Part model, mm, in its own coordinate system. Face numbers are marked on the shaded views. Round coordinates to 2 decimals unless told otherwise and drop trailing zeros. Loops run counter-clockwise (first coordinate to the right, second up) from the corner with the lowest first, then second, coordinate; pieces in that order, holes last.
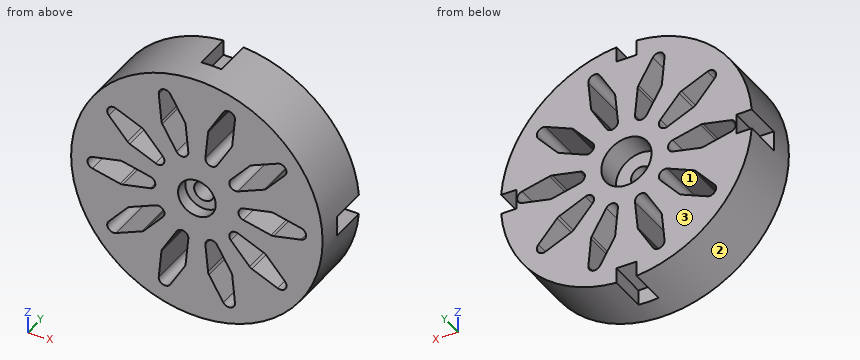
from build123d import *

# Parameters (mm, degrees)
SKETCH_1_R               = 20
SKETCH_1_R_2             = 4
EXTRUDE_1_DEPTH          = 10
SKETCH_4_R               = 20
EXTRUDE_2_DEPTH          = 6
SKETCH_5_R               = 1.6
CUT_EXTRUDE_2_DEPTH      = 5
CUT_EXTRUDE_2_DEPTH_BACK = 7
CUT_EXTRUDE_3_DEPTH      = 1
CUT_EXTRUDE_3_DEPTH_BACK = 11
SKETCH_8_W               = 3.2
SKETCH_8_H               = 5
SKETCH_8_W_2             = 5
SKETCH_8_H_2             = 3.2
CUT_EXTRUDE_4_DEPTH      = 6
SKETCH_9_R               = 3
CUT_EXTRUDE_5_DEPTH      = 2


with BuildPart() as part:
    # Эскиз1 → Бобышка-Вытянуть1 (new body)
    with BuildSketch(Plane(origin=(0, 0, 0), x_dir=(1, 0, 0), z_dir=(0, 1, 0))):
        Circle(SKETCH_1_R)
        Circle(SKETCH_1_R_2, mode=Mode.SUBTRACT)
    extrude(amount=EXTRUDE_1_DEPTH)

    # Эскиз4 → Бобышка-Вытянуть2 (add)
    with BuildSketch(Plane.XZ):
        Circle(SKETCH_4_R)
    extrude(amount=-EXTRUDE_2_DEPTH)

    # Эскиз5 → Вырез-Вытянуть2 (cut, two sides)
    with BuildSketch(Plane(origin=(0, 6, 0), x_dir=(1, 0, 0), z_dir=(0, 1, 0))) as cut_extrude_2_sk:
        Circle(SKETCH_5_R)
    extrude(amount=CUT_EXTRUDE_2_DEPTH, mode=Mode.SUBTRACT)
    extrude(cut_extrude_2_sk.sketch, amount=-CUT_EXTRUDE_2_DEPTH_BACK, mode=Mode.SUBTRACT)

    # Эскиз6 → Вырез-Вытянуть3 (cut, two sides)
    with BuildSketch(Plane.XZ) as cut_extrude_3_sk:
        with BuildLine():
            Line((-7.392841771, 0.97618706), (-11.783069542, 1.951793232))
            ThreePointArc((-11.783069542, 1.951793232), (-12, 1.975606171), (-12.216930458, 1.951793232))
            Line((-12.216930458, 1.951793232), (-16.607158229, 0.97618706))
            ThreePointArc((-16.607158229, 0.97618706), (-17.390227771, 0), (-16.607158229, -0.97618706))
            Line((-16.607158229, -0.97618706), (-12.216930458, -1.951793232))
            ThreePointArc((-12.216930458, -1.951793232), (-12, -1.975606171), (-11.783069542, -1.951793232))
            Line((-11.783069542, -1.951793232), (-7.392841771, -0.97618706))
            ThreePointArc((-7.392841771, -0.97618706), (-6.609772229, 0), (-7.392841771, 0.97618706))
        make_face()
        with BuildLine():
            Line((-5.407146272, 5.135155287), (-8.385468228, 8.504948397))
            ThreePointArc((-8.385468228, 8.504948397), (-8.546971761, 8.651721994), (-8.736469082, 8.759965445))
            Line((-8.736469082, 8.759965445), (-12.861684878, 10.551194611))
            ThreePointArc((-12.861684878, 10.551194611), (-14.068989803, 10.221719418), (-14.009261593, 8.971690768))
            Line((-14.009261593, 8.971690768), (-11.030939637, 5.601897658))
            ThreePointArc((-11.030939637, 5.601897658), (-10.869436104, 5.455124061), (-10.679938783, 5.34688061))
            Line((-10.679938783, 5.34688061), (-6.554722987, 3.555651444))
            ThreePointArc((-6.554722987, 3.555651444), (-5.347418062, 3.885126637), (-5.407146272, 5.135155287))
        make_face()
        with BuildLine():
            Line((-1.356104679, 7.332668731), (-1.784903063, 11.809502348))
            ThreePointArc((-1.784903063, 11.809502348), (-1.82929081, 12.023174077), (-1.918973459, 12.222128599))
            Line((-1.918973459, 12.222128599), (-4.203485056, 16.096004442))
            ThreePointArc((-4.203485056, 16.096004442), (-5.373875917, 16.539089442), (-6.060303186, 15.49268766))
            Line((-6.060303186, 15.49268766), (-5.631504802, 11.015854043))
            ThreePointArc((-5.631504802, 11.015854043), (-5.587117055, 10.802182314), (-5.497434406, 10.603227792))
            Line((-5.497434406, 10.603227792), (-3.212922809, 6.729351949))
            ThreePointArc((-3.212922809, 6.729351949), (-2.042531948, 6.286266949), (-1.356104679, 7.332668731))
        make_face()
        with BuildLine():
            Line((3.212922809, 6.729351949), (5.497434406, 10.603227792))
            ThreePointArc((5.497434406, 10.603227792), (5.587117055, 10.802182314), (5.631504802, 11.015854043))
            Line((5.631504802, 11.015854043), (6.060303186, 15.49268766))
            ThreePointArc((6.060303186, 15.49268766), (5.373875917, 16.539089442), (4.203485056, 16.096004442))
            Line((4.203485056, 16.096004442), (1.918973459, 12.222128599))
            ThreePointArc((1.918973459, 12.222128599), (1.82929081, 12.023174077), (1.784903063, 11.809502348))
            Line((1.784903063, 11.809502348), (1.356104679, 7.332668731))
            ThreePointArc((1.356104679, 7.332668731), (2.042531948, 6.286266949), (3.212922809, 6.729351949))
        make_face()
        with BuildLine():
            Line((6.554722987, 3.555651444), (10.679938783, 5.34688061))
            ThreePointArc((10.679938783, 5.34688061), (10.869436104, 5.455124061), (11.030939637, 5.601897658))
            Line((11.030939637, 5.601897658), (14.009261593, 8.971690768))
            ThreePointArc((14.009261593, 8.971690768), (14.068989803, 10.221719418), (12.861684878, 10.551194611))
            Line((12.861684878, 10.551194611), (8.736469082, 8.759965445))
            ThreePointArc((8.736469082, 8.759965445), (8.546971761, 8.651721994), (8.385468228, 8.504948397))
            Line((8.385468228, 8.504948397), (5.407146272, 5.135155287))
            ThreePointArc((5.407146272, 5.135155287), (5.347418062, 3.885126637), (6.554722987, 3.555651444))
        make_face()
        with BuildLine():
            Line((7.392841771, -0.97618706), (11.783069542, -1.951793232))
            ThreePointArc((11.783069542, -1.951793232), (12, -1.975606171), (12.216930458, -1.951793232))
            Line((12.216930458, -1.951793232), (16.607158229, -0.97618706))
            ThreePointArc((16.607158229, -0.97618706), (17.390227771, 0), (16.607158229, 0.97618706))
            Line((16.607158229, 0.97618706), (12.216930458, 1.951793232))
            ThreePointArc((12.216930458, 1.951793232), (12, 1.975606171), (11.783069542, 1.951793232))
            Line((11.783069542, 1.951793232), (7.392841771, 0.97618706))
            ThreePointArc((7.392841771, 0.97618706), (6.609772229, 0), (7.392841771, -0.97618706))
        make_face()
        with BuildLine():
            Line((5.407146272, -5.135155287), (8.385468228, -8.504948397))
            ThreePointArc((8.385468228, -8.504948397), (8.546971761, -8.651721994), (8.736469082, -8.759965445))
            Line((8.736469082, -8.759965445), (12.861684878, -10.551194611))
            ThreePointArc((12.861684878, -10.551194611), (14.068989803, -10.221719418), (14.009261593, -8.971690768))
            Line((14.009261593, -8.971690768), (11.030939637, -5.601897658))
            ThreePointArc((11.030939637, -5.601897658), (10.869436104, -5.455124061), (10.679938783, -5.34688061))
            Line((10.679938783, -5.34688061), (6.554722987, -3.555651444))
            ThreePointArc((6.554722987, -3.555651444), (5.347418062, -3.885126637), (5.407146272, -5.135155287))
        make_face()
        with BuildLine():
            Line((1.356104679, -7.332668731), (1.784903063, -11.809502348))
            ThreePointArc((1.784903063, -11.809502348), (1.82929081, -12.023174077), (1.918973459, -12.222128599))
            Line((1.918973459, -12.222128599), (4.203485056, -16.096004442))
            ThreePointArc((4.203485056, -16.096004442), (5.373875917, -16.539089442), (6.060303186, -15.49268766))
            Line((6.060303186, -15.49268766), (5.631504802, -11.015854043))
            ThreePointArc((5.631504802, -11.015854043), (5.587117055, -10.802182314), (5.497434406, -10.603227792))
            Line((5.497434406, -10.603227792), (3.212922809, -6.729351949))
            ThreePointArc((3.212922809, -6.729351949), (2.042531948, -6.286266949), (1.356104679, -7.332668731))
        make_face()
        with BuildLine():
            Line((-3.212922809, -6.729351949), (-5.497434406, -10.603227792))
            ThreePointArc((-5.497434406, -10.603227792), (-5.587117055, -10.802182314), (-5.631504802, -11.015854043))
            Line((-5.631504802, -11.015854043), (-6.060303186, -15.49268766))
            ThreePointArc((-6.060303186, -15.49268766), (-5.373875917, -16.539089442), (-4.203485056, -16.096004442))
            Line((-4.203485056, -16.096004442), (-1.918973459, -12.222128599))
            ThreePointArc((-1.918973459, -12.222128599), (-1.82929081, -12.023174077), (-1.784903063, -11.809502348))
            Line((-1.784903063, -11.809502348), (-1.356104679, -7.332668731))
            ThreePointArc((-1.356104679, -7.332668731), (-2.042531948, -6.286266949), (-3.212922809, -6.729351949))
        make_face()
        with BuildLine():
            Line((-6.554722987, -3.555651444), (-10.679938783, -5.34688061))
            ThreePointArc((-10.679938783, -5.34688061), (-10.869436104, -5.455124061), (-11.030939637, -5.601897658))
            Line((-11.030939637, -5.601897658), (-14.009261593, -8.971690768))
            ThreePointArc((-14.009261593, -8.971690768), (-14.068989803, -10.221719418), (-12.861684878, -10.551194611))
            Line((-12.861684878, -10.551194611), (-8.736469082, -8.759965445))
            ThreePointArc((-8.736469082, -8.759965445), (-8.546971761, -8.651721994), (-8.385468228, -8.504948397))
            Line((-8.385468228, -8.504948397), (-5.407146272, -5.135155287))
            ThreePointArc((-5.407146272, -5.135155287), (-5.347418062, -3.885126637), (-6.554722987, -3.555651444))
        make_face()
    extrude(amount=CUT_EXTRUDE_3_DEPTH, mode=Mode.SUBTRACT)
    extrude(cut_extrude_3_sk.sketch, amount=-CUT_EXTRUDE_3_DEPTH_BACK, mode=Mode.SUBTRACT)

    # Эскиз8 → Вырез-Вытянуть4 (cut)
    with BuildSketch(Plane(origin=(0, 10, 0), x_dir=(1, 0, 0), z_dir=(0, 1, 0))):
        with Locations((0, 20)):
            Rectangle(SKETCH_8_W, SKETCH_8_H)
        with Locations((-20, 0)):
            Rectangle(SKETCH_8_W_2, SKETCH_8_H_2)
        with Locations((20, 0)):
            Rectangle(SKETCH_8_W_2, SKETCH_8_H_2)
        with Locations((0, -20)):
            Rectangle(SKETCH_8_W, SKETCH_8_H)
    extrude(amount=-CUT_EXTRUDE_4_DEPTH, mode=Mode.SUBTRACT)

    # Эскиз9 → Вырез-Вытянуть5 (cut)
    with BuildSketch(Plane.XZ):
        Circle(SKETCH_9_R)
    extrude(amount=-CUT_EXTRUDE_5_DEPTH, mode=Mode.SUBTRACT)


solid = part.part
1) Slice it at B-B, the plane z = 0. Give the cut face in (x, y), then the cut area to 3 significant figures.
Values:
outline: (-20, 0) - (-17.39, 0) - (-17.39, 10) - (-17.5, 10) - (-17.5, 4) - (-20, 4) - close; (-6.61, 0) - (-3, 0) - (-3, 2) - (-1.6, 2) - (-1.6, 6) - (-4, 6) - (-4, 10) - (-6.61, 10) - close; (1.6, 2) - (3, 2) - (3, 0) - (6.61, 0) - (6.61, 10) - (4, 10) - (4, 6) - (1.6, 6) - close; (17.39, 0) - (20, 0) - (20, 4) - (17.5, 4) - (17.5, 10) - (17.39, 10) - close
area: 97.6 mm2
2) Wall check: line 1 along Z through (x, y) = (0, 4.2); line 2 along Z through (x, y) = (0, 0.85); line 3 along X through (y, z) = (4.5, -12). Give the ranges that are in metal, low to high.
Values:
line 1: z = -17.5 to -1.6, 1.6 to 17.5
line 2: z = -20 to -3, 3 to 20
line 3: x = -16 to -5.73, -1.82 to 1.82, 5.73 to 16
3) Slice it at C-C, the plane z = 13. Give the cut face in (x, y), then the cut area to 3 significant figures.
Values:
outline: (-15.2, 0) - (-5.82, 0) - (-5.82, 10) - (-15.2, 10) - close; (-2.38, 0) - (2.38, 0) - (2.38, 10) - (-2.38, 10) - close; (5.82, 0) - (15.2, 0) - (15.2, 10) - (5.82, 10) - close
area: 235 mm2
4) Mould opens along X. For the marked faces 1, 2 and 3 say: released by +X, released by -X, zero draft, split by the parting line, or undercut.
Values:
face 1: undercut
face 2: split by the parting line
face 3: zero draft
5) Slice it at A-A, the plane x = 0. Give the cut face in (y, z).
Values:
outline: (0, -20) - (4, -20) - (4, -17.5) - (10, -17.5) - (10, -4) - (6, -4) - (6, -1.6) - (2, -1.6) - (2, -3) - (0, -3) - close; (0, 3) - (2, 3) - (2, 1.6) - (6, 1.6) - (6, 4) - (10, 4) - (10, 17.5) - (4, 17.5) - (4, 20) - (0, 20) - close
6) Slice it at D-D, the plane x = 15. Give the cut face in (y, z).
Values:
outline: (0, -13.23) - (10, -13.23) - (10, -1.33) - (0, -1.33) - close; (0, 1.33) - (10, 1.33) - (10, 13.23) - (0, 13.23) - close
7) Drop flat-ended pins along their axis: pin 1 Ø0.7 at (y, z) = (7.5, -18.5) entering from -X; pin 2 Ø2.5 at (x, y) = (18, 5.5) entering from -Z; pin 3 Ø5 at (x, y) = (-15, 3) entering from -Z; pin 4 Ø2.5 at (x, z) = (0, 0) entering from +Y. Give the stop position or say it passes through.
Values:
pin 1: stops at x = -8.4
pin 2: stops at z = -10.93
pin 3: stops at z = -15.61
pin 4: passes through
